Autodesk Inventor part; units mm, degrees
ref_plane "YZ Plane" through (0, 0, 0) normal (1, 0, 0) x (0, 1, 0)
ref_plane "XZ Plane" through (0, 0, 0) normal (0, 1, 0) x (-1, 0, 0)
ref_plane "XY Plane" through (0, 0, 0) normal (0, 0, 1) x (1, 0, 0)
sketch "Boceto1" plane through (0, 0, 0) normal (0, 1, 0) x (-1, 0, 0)
  circle A0 centre (1.5044, -21.0374) radius 7
  line L0 (0, 0) -> (-30, 0) construction
  line L1 (0, 0) -> (35.019, 45) construction
  arc A1 (45.0717, 45) -> (29.0132, 53.0615) centre (35.019, 45) ccw
  arc A2 (28.1996, -43.444) -> (39.4639, -39.5994) centre (35.019, -45) ccw
  arc A3 (29.0141, -53.0621) -> (45.0717, -45) centre (35.019, -45) ccw
  line L2 (45.0717, 45) -> (45.0717, -45)
  line L3 (-31.4523, -8.0252) -> (29.0141, -53.0621)
  line L4 (-31.4532, 8.0139) -> (29.0132, 53.0615)
  circle A4 centre (35.019, -45) radius 2.5
  line L5 (35.019, 45) -> (35.019, -45) construction
  line L6 (0, 0) -> (35.019, -45) construction
  arc A5 (39.4623, 39.5898) -> (28.1951, 43.4351) centre (35.019, 45) ccw
  line L7 (37.5264, -35.4953) -> (37.5264, 35.4947)
  line L8 (32.5115, -34.8171) -> (32.5115, 34.8171)
  line L9 (4.23, 5.4356) -> (6.2005, 3.9021) construction
  line L10 (7.7468, 5.9499) -> (30.7228, 35.4318)
  line L11 (3.8646, 8.971) -> (27.2206, 39.0273)
  line L12 (7.7468, -5.9499) -> (30.7228, -35.4318)
  line L13 (3.8646, -8.971) -> (27.2206, -39.0273)
  arc A6 (32.5115, 34.8171) -> (30.7228, 35.4318) centre (31.5115, 34.8171) ccw
  arc A7 (30.7228, -35.4318) -> (32.5115, -34.8171) centre (31.5115, -34.8171) ccw
  arc A8 (27.2206, 39.0273) -> (28.1951, 43.4351) centre (23.063, 42.2581) ccw
  arc A9 (-0.1798, 6.8852) -> (3.8646, 8.971) centre (-0.4077, 12.2909) ccw
  arc A10 (7.7468, 5.9499) -> (6.7608, 1.532) centre (11.9166, 2.7002) ccw
  arc A11 (6.7608, -1.532) -> (7.7468, -5.9499) centre (11.9166, -2.7002) ccw
  arc A12 (3.8646, -8.971) -> (-0.1798, -6.8852) centre (-0.4077, -12.2909) ccw
  arc A13 (6.7608, -1.532) -> (6.7608, 1.532) centre (0, 0) ccw
  arc A14 (-0.1798, 6.8852) -> (-0.1798, -6.8852) centre (0, 0) ccw
  arc A15 (39.4623, 39.5898) -> (37.5264, 35.4947) centre (42.8256, 35.4947) ccw
  arc A16 (37.5264, -35.4953) -> (39.4639, -39.5994) centre (42.8417, -35.4953) ccw
  arc A17 (28.1996, -43.444) -> (27.2206, -39.0273) centre (23.0492, -42.2688) ccw
  arc A18 (-31.4532, 8.0139) -> (-31.4523, -8.0252) centre (-25.4789, -0.0053) ccw
  line L14 (29.0115, 27.5422) -> (29.0115, -27.5422)
  line L15 (29.0115, -27.5422) -> (10.5075, -3.7984)
  arc A19 (10.1743, -2.3054) -> (10.5075, -3.7984) centre (11.9166, -2.7002) ccw
  arc A20 (10.1743, -2.3054) -> (10.1743, 2.3054) centre (0, 0) ccw
  arc A21 (10.5075, 3.7984) -> (10.1743, 2.3054) centre (11.9166, 2.7002) ccw
  line L16 (10.5075, 3.7984) -> (29.0115, 27.5422)
  line L17 (39.5264, 35.8019) -> (39.5264, -35.8019)
  line L18 (40.8447, 38.0421) -> (40.8447, -38.1418) construction
  line L19 (21.3809, 43.6361) -> (-23.936, 9.8749)
  arc A22 (23.8235, 40.3575) -> (21.3809, 43.6361) centre (22.6022, 41.9968) ccw
  arc A23 (-1.3686, 9.7923) -> (-9.8875, 0) centre (0, 0) ccw
  line L20 (23.8235, 40.3575) -> (1.2488, 11.3067)
  arc A24 (-1.3686, 9.7923) -> (1.2488, 11.3067) centre (-1.9249, 13.773) ccw
  arc A25 (-29.6624, 5.6176) -> (-29.9588, -5.3847) centre (-25.486, 0) ccw
  line L21 (-23.936, 9.8749) -> (-29.6624, 5.6176)
  arc A26 (-9.8875, 0) -> (-1.8786, -9.7074) centre (0, 0) ccw
  line L22 (43.1749, 35.8019) -> (43.1749, -35.8019)
  arc A27 (43.1749, 35.8019) -> (39.5264, 35.8019) centre (41.3506, 35.8019) ccw
  arc A28 (39.5264, -35.8019) -> (43.1749, -35.8019) centre (41.3506, -35.8019) ccw
  line L23 (-30, -5.3501) -> (-8.2939, -21.5174)
  arc A29 (2.552, -11.1194) -> (-1.8786, -9.7074) centre (-5.6513, -29.2032) ccw
  arc A30 (2.3012, -12.0728) -> (2.552, -11.1194) centre (2.3454, -11.5747) ccw
  arc A31 (-8.2939, -21.5174) -> (-7.4953, -21.1122) centre (-7.9953, -21.1164) ccw
  line L24 (11.2288, -22.5221) -> (24.908, -40.1255)
  line L25 (3.8504, -30.5629) -> (21.4406, -43.6644)
  arc A32 (21.4406, -43.6644) -> (24.908, -40.1255) centre (22.9339, -41.6595) ccw
  arc A33 (2.3012, -12.0728) -> (-2.6092, -13.0325) centre (1.5044, -21.0374) ccw
  arc A34 (-5.1216, -14.9468) -> (-7.4953, -21.1122) centre (1.5044, -21.0374) ccw
  arc A35 (2.3012, -12.0728) -> (-7.4953, -21.1122) centre (1.5044, -21.0374) ccw
  arc A36 (4.0099, -29.6816) -> (10.3429, -22.7346) centre (1.5044, -21.0374) ccw
  arc A37 (11.2288, -22.5221) -> (10.3429, -22.7346) centre (10.834, -22.8289) ccw
  arc A38 (4.0099, -29.6816) -> (3.8504, -30.5629) centre (4.1491, -30.1619) ccw
  point P0 (31.1449, 35.9734)
  point P1 (32.5115, 35.4947)
  point P2 (32.5115, -35.4953)
  point P3 (32.5115, 35.4947)
  point P4 (31.1449, -35.9734)
  point P5 (-3.2933, -26.1347)
  point P6 (8.3262, -19.468)
  point P7 (-7.4247, -22.1648)
  point P8 (10.4887, -21.5697)
  point P9 (2.9812, -29.9154)
  point P10 (-2.6092, -13.0325)
  dimension "d0" = 14
  dimension "d1" = 45
  dimension "d2" = 5
  dimension "d3" = 1
  dimension "d4" = 10
  dimension "d5" = 3.5
  dimension "d6" = 2
  dimension "d7" = 3
  dimension "d8" = 14
  dimension "d20" = 0.5
  dimension "d23" = 2.5
  dimension "d24" = 2.5
  dimension "d25" = 0.5
extrude "Extrusión2" add sketch "Boceto1" along normal blind 5 contours A0 | A17 L13 A12 A14 A9 L11 A8 A5 A15 L7 A16 A2
extrude "Extrusión3" add sketch "Boceto1" along normal blind 15 contours A4
extrude "Extrusión4" add sketch "Boceto1" along normal blind 3 contours L2 A3 L3 A18 L4 A1
extrude "Extrusión5" add sketch "Boceto1" along normal blind 3 contours A7 L12 A11 A13 A10 L10 A6 L8
sketch "Boceto2" plane through (-35.019, 15, -45) normal (0, 1, 0) x (1, 0, 0)
  circle A0 centre (0, 0) radius 7
  point P0 (35.019, -45)
  dimension "d30" = 14
extrude "Extrusión6" add sketch "Boceto2" along normal blind 2
fillet "Empalme1" radius 2 1 edges at (-32.519, 15, -45)
fillet "Empalme2" radius 1 1 edges at (-42.019, 15, -45)
properties part number "prot2"
For this review, take the finished solid that the model builds, in its own axes (mm). A direction names the side the tool comes from. Coordinates: 2 decimals unless noted, no trailing zeros. Loops run counter-clockwise (first coordinate to the right, second up) from the corner with the lowest first, then second, coordinate; pieces in that order, holes last. Notation, with made-up numbers: (20.25, 2.5) - (69.25, 2.5) arc R35 ccw to (69.25, 35.5) - close; hole circle Ø1 at (-29.75, -26.5). An arc over 180 degrees is marked (long way). Use one line per item in the form item = value. Start each with the question number.
1) For faces 5 (the face through (-17.97, 1.48, -31.2)), 6 (the face through (35.478, 1.479, -0.136)), 7 (the face through (0, 4, -14.2)), 8 (the face through (-36.4, 15, -49.5)), list the 3-axis set-ups (+Z, -Z, +X, -X, +Y, -Y) from which the entire face can be reached by the end or side of a thin tool; tool diameter is ignored.
2) For pin 1 (11 mm diameter, centred on x = 1, z = -22, fed in from +Y); pin 2 (5 mm diameter, centred on x = -26, y = 3.5, fed in from -Z); pin 3 (0.9 mm diameter, centred on y = 2, z = 12.5, fed in from +X), all flat-tipped, find the tip position at first contact; note any pin that passes through.
3) Take a section at A-A (x = -13). State the section outline as (y, z) points.
4) To check wall thickness, follow probe 1 along Y at (x, z) = (-11, 12); probe 2 along Y at (x, z) = (-38, 3); probe 3 along Y at (x, z) = (-32.5, -48). State the ranges of each line that lie inside material, in increasing order. Write a range as from..to.
5) Draft analysis for pull direction Z (two halves, no side actions). For faces 1 (the face through (-2.102, 3.986, 7.497)), 2 (the face through (-41.391, 1.479, -37.626)), 3 (the face through (-30, 3, 3)), 4 (the face through (-35.93, 16.49, -38.06)), state which applies: released by +Z, released by -Z, zero draft, split by the parting line, or undercut.
6) Take a section at B-B (y = 7). State the section outline as (x, z) points, plus the area to 3 significant figures.
From the geometry:
q1.face_5 = +Y, -Y
q1.face_6 = +X, +Y, -Y
q1.face_7 = +Y
q1.face_8 = none
q2.pin_1 = 5
q2.pin_2 = -52.64
q2.pin_3 = 26.04
q3.outline = (0, -41.13) - (3, -41.13) - (3, -37.38) - (0, -37.38) - close; (0, -24.8) - (3, -24.8) - (3, -20.73) - (5, -20.73) - (5, -12.69) - (3, -12.69) - (3, -7) - (0, -7) - close; (0, 7) - (3, 7) - (3, 12.69) - (5, 12.69) - (5, 20.73) - (3, 20.73) - (3, 26.43) - (0, 26.43) - close; (0, 37.39) - (3, 37.39) - (3, 41.13) - (0, 41.13) - close
q4.probe_1 = 0..5
q4.probe_2 = 0..3
q4.probe_3 = 0..5, 14.91..17
q5.face_1 = released by +Z
q5.face_2 = undercut
q5.face_3 = undercut
q5.face_4 = split by the parting line
q6.outline = circle Ø5 at (-35.02, -45)
q6.area = 19.6 mm2
